Geometry: final body of the model. Coordinates: model frame, mm. A direction names the side the tool comes from. Give positions to 0.01 mm unless a question says otherwise; leave off trailing zeros. Order: outer loops, then holes, each group sorted by start corner. A loop starts at its lowest first (then second) coordinate and runs counter-clockwise, first axis right, second up. Notation, with made-up numbers: (21.5, 18) - (38.5, 18) arc R13 ccw to (38.5, 28) - close; hole circle Ø6 at (14, 40.5). An arc over 180 degrees is marked (long way). Write item = value, one per line. Start each with the question number.
from build123d import *

# Parameters (mm, degrees)
F1_DEPTH    = 6.35
F2_W        = 2.8327330947
F2_H        = 10.4811154306
F3_DEPTH    = 3.175
F4_T4_DEPTH = 134.7141247892
F6_DEPTH    = 6.35


# Not quite as in the source:
# - a fillet or chamfer that OpenCascade refuses, or shapes differently, is made with other operations: its cross-section is extruded or revolved along the edge and cut away or added
# - a feature names something its author has since deleted; it is built from what else it names


with BuildPart() as f1:
    # F0 (on Front) → F1 (new body, symmetric)
    with BuildSketch(Plane.XZ):
        with BuildLine():
            Line((17.3079642735, 0), (17.3079642735, 25.4))
            Line((17.3079642735, 25.4), (-33.4920357265, 0))
            Line((-33.4920357265, 0), (-27.5403555314, 0))
            ThreePointArc((-27.5403555314, 0), (-23.9862389863, 3.5541165451), (-20.4321224411, 0))
            Line((-20.4321224411, 0), (5.2073936615, 0))
            ThreePointArc((5.2073936615, 0), (8.7613936615, 3.554), (12.3153936615, 0))
            Line((12.3153936615, 0), (17.3079642735, 0))
        make_face()
    extrude(amount=F1_DEPTH, both=True)

    # F2 (on Front) → F3 (join, symmetric)
    with BuildSketch(Plane.XZ):
        with Locations((-24.0782387555, 5.2405577153)):
            Rectangle(F2_W, F2_H)
        with Locations((8.7149282917, 5.2405577153)):
            Rectangle(F2_W, F2_H)
    extrude(amount=F3_DEPTH, both=True)

    # F4: fillet of radius 54.0783837972 on 1 edges, made by hand


with BuildPart() as f4_tool2:
    # F4_s3 → F4_t4 (new body)
    with BuildSketch(Plane.XZ.offset(-67.3570623946)):
        with BuildLine():
            ThreePointArc((-25.4946053028, 3.9987152119), (-13.0610727535, 8.8354764656), (0.178219655, 10.4811154306))
            Line((0.178219655, 10.4811154306), (-25.4946053028, 10.4811154306))
            Line((-25.4946053028, 10.4811154306), (-25.4946053028, 3.9987152119))
        make_face()
    extrude(amount=F4_T4_DEPTH)

    split(bisect_by=Plane.YZ.offset(-22.6618722081), keep=Keep.BOTTOM)


with BuildPart() as f1_1:
    add(f1.part)

    # F4_t1: cut F4_tool2
    add(f4_tool2.part, mode=Mode.SUBTRACT)

    # F5 (on Front) → F6 (join, symmetric)
    with BuildSketch(Plane.XZ):
        with BuildLine():
            ThreePointArc((-25.4952833056, 0), (-24.0811295807, -1.4141537249), (-22.6669758558, 0))
            ThreePointArc((-22.6669758558, 0), (-24.0811295807, 1.4141537249), (-25.4952833056, 0))
        make_face()
        with BuildLine():
            ThreePointArc((7.2927195579, 0), (8.7104998529, -1.4270738296), (10.1282801479, 0))
            ThreePointArc((10.1282801479, 0), (8.7104998529, 1.417780295), (7.2927195579, 0))
        make_face()
    extrude(amount=F6_DEPTH, both=True)


solid = f1_1.part
Q1. Section A-A, the plane y = 4. Return the cut outline in (x, z), then the cut area to 3 significant figures.
Q2. Section C-C, the plane z = 20.5. Return the cut outline in (x, y), then the cut area to 3 significant figures.
Q3. Material intervals for line 1 along X through (y, z) = (1.5, 0.25); line 2 along Z through (x, y) = (9.5, -3.75); line 3 along X through (y, z) = (2.25, 22.5), sorted ascending. Write a range as from..to.
Q4. Contact query for flat-ended pins moving along their axis: pin 1 (3 mm diameter, centred on x = -2, y = 5, fed in from -Z); pin 2 (2.5 mm diameter, centred on x = -23.5, z = 2, fed in from -Y); pin 3 (0.9 mm diameter, centred on y = 0, z = 1, fed in from -X); pin 4 (1 mm diameter, centred on x = -14, y = 2, fed in from +Z). Output: stop coordinate, or through.
Q5. Pull-direction query (X, two-part tool) for faces 5 (the flat face through (3, -6.35, 7)), 6 (the flat face through (10.131, 0, 2)), 7 (the flat face through (17.308, 0, 13)); classes: +X half, -X half, draft (parallel to the pull), parting line (faces both ways), or undercut.
Q6. Set-up query: faces 1 (the flat face through (7.299, 0, 2)), 2 (the flat face through (15, 0, 0)), 3 (the cylindrical face through (8.742, -4.322, 1.417)), 4 (the flat face through (-24, 3.175, 2)). Return all of +Z, -Z, +X, -X, +Y, -Y with unobstructed straight access to the full face (end or side cutting, diameter ignored); none if empty.
Q7. Section D-D, the plane x = -7. Return the cut outline in (y, z), then the cut area to 3 significant figures.
The answers:
q1.outline = (-33.49, 0) - (-27.54, 0) arc R3.55 cw to (-20.43, 0) - (5.21, 0) arc R3.55 cw to (12.32, 0) - (17.31, 0) - (17.31, 25.4) - close; circle Ø2.83 at (-24.08, 0); (7.29, 0) arc R1.42 ccw (long way) to (10.13, 0) arc R1.42 ccw to start
q1.area = 618 mm²
q2.outline = (7.51, -6.35) - (17.31, -6.35) - (17.31, 6.35) - (7.51, 6.35) - close
q2.area = 124 mm²
q3.line_1 = -32.99..-27.53, -25.49..-22.66, -20.44..5.22, 7.3..10.13, 12.31..17.31
q3.line_2 = -1.19..1.18, 3.48..21.5
q3.line_3 = 11.51..17.31
q4.pin_1 = 0
q4.pin_2 = -6.35
q4.pin_3 = -32.39
q4.pin_4 = 10
q5.face_5 = draft
q5.face_6 = undercut
q5.face_7 = +X half
q6.face_1 = -Z, +Y, -Y
q6.face_2 = -Z, +X, +Y, -Y
q6.face_3 = none
q6.face_4 = +Y
q7.outline = (-6.35, 0) - (6.35, 0) - (6.35, 13.25) - (-6.35, 13.25) - close
q7.area = 168 mm²
